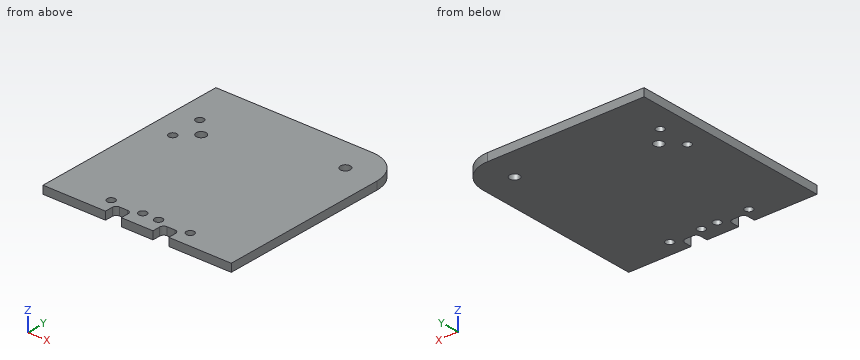
```python
from build123d import *

# Parameters (mm, degrees)
SKETCH_1_R      = 1.25
SKETCH_1_R_2    = 1
EXTRUDE_2_DEPTH = 2


with BuildPart() as part:
    # 草圖1 → 填料-伸長2 (new body)
    with BuildSketch(Plane.XY):
        with BuildLine():
            Line((-28.541905067, -5.335177429), (-28.541905067, -52.335177429))
            Line((-28.541905067, -52.335177429), (-28.541905067, -53.6179941))
            Line((-28.541905067, -53.6179941), (-28.541905067, -55.6179941))
            Line((-28.541905067, -55.6179941), (-12.741905067, -55.6179941))
            Line((-12.741905067, -55.6179941), (-12.741905067, -53.6179941))
            ThreePointArc((-12.741905067, -53.6179941), (-12.449011848, -52.910887319), (-11.741905067, -52.6179941))
            Line((-11.741905067, -52.6179941), (-9.741905067, -52.6179941))
            ThreePointArc((-9.741905067, -52.6179941), (-9.034798286, -52.910887319), (-8.741905067, -53.6179941))
            Line((-8.741905067, -53.6179941), (-8.741905067, -55.6179941))
            Line((-8.741905067, -55.6179941), (-0.741905067, -55.6179941))
            Line((-0.741905067, -55.6179941), (-0.741905067, -53.6179941))
            ThreePointArc((-0.741905067, -53.6179941), (-0.449011848, -52.910887319), (0.258094933, -52.6179941))
            Line((0.258094933, -52.6179941), (2.258094933, -52.6179941))
            ThreePointArc((2.258094933, -52.6179941), (2.965201714, -52.910887319), (3.258094933, -53.6179941))
            Line((3.258094933, -53.6179941), (3.258094933, -55.6179941))
            Line((3.258094933, -55.6179941), (19.058094933, -55.6179941))
            Line((19.058094933, -55.6179941), (19.058094933, -53.900810772))
            Line((19.058094933, -53.900810772), (19.058094933, -52.6179941))
            Line((19.058094933, -52.6179941), (19.058094933, -12.6179941))
            ThreePointArc((19.058094933, -12.6179941), (16.714949182, -6.961139851), (11.058094933, -4.6179941))
            Line((11.058094933, -4.6179941), (-27.541905067, -4.6179941))
            Line((-27.541905067, -4.6179941), (-28.541905067, -4.6179941))
            Line((-28.541905067, -4.6179941), (-28.541905067, -5.335177429))
        make_face()
        with Locations((-18.541905067, -20.6179941)):
            Circle(SKETCH_1_R, mode=Mode.SUBTRACT)
        with Locations((-6.741905067, -51.6179941)):
            Circle(SKETCH_1_R_2, mode=Mode.SUBTRACT)
        with Locations((-22.541905067, -16.3679941)):
            Circle(SKETCH_1_R_2, mode=Mode.SUBTRACT)
        with Locations((-22.541905067, -24.3679941)):
            Circle(SKETCH_1_R_2, mode=Mode.SUBTRACT)
        with Locations((11.058094933, -12.6179941)):
            Circle(SKETCH_1_R, mode=Mode.SUBTRACT)
        with Locations((-14.741905067, -51.6179941)):
            Circle(SKETCH_1_R_2, mode=Mode.SUBTRACT)
        with Locations((5.258094933, -51.6179941)):
            Circle(SKETCH_1_R_2, mode=Mode.SUBTRACT)
        with Locations((-2.741905067, -51.6179941)):
            Circle(SKETCH_1_R_2, mode=Mode.SUBTRACT)
    extrude(amount=EXTRUDE_2_DEPTH)


solid = part.part
```
Verification items for the finished model (mm, model axes). Give positions to 0.01 mm unless a question says otherwise; leave off trailing zeros. Answer as CSV lines item,"result". Start each with the question number.
Item 1: Section check A-A, the plane z = 0.6. State how many separate pieces and enclosed holes the cut face has, plus the area to 3 significant figures.
Item 2: Material ranges on L1, parallel to Y at x = -22.5, z = 1; L2, parallel to X at y = -51.5, z = 0.2; L3, parallel to Y at x = -10, z = 0.45, recorded low to high.
Item 3: Gauge pin test, flat end, axial feed: pin 1 (1 mm diameter, centred on x = -10.5, z = 1, fed in from -Y). Record the tip position at first contact, or that the pin passes through.
Filled in:
1,separate pieces,"1"
1,enclosed holes,"8"
1,area,"2,360 mm^2"
2,L1,"-55.62 to -25.37, -23.37 to -17.37, -15.37 to -4.62"
2,L2,"-28.54 to -15.73, -13.75 to -7.73, -5.75 to -3.73, -1.75 to 4.27, 6.25 to 19.06"
2,L3,"-52.62 to -4.62"
3,pin 1,"y = -52.62"
